from build123d import *

# Parameters (mm, degrees)
SKETCH1_R                           = 12.5
BOSS_EXTRUDE1_DEPTH                 = 50
CUT_EXTRUDE1_REACH                  = 55.033
CUT_EXTRUDE1_END_RADIUS             = 12.5
SKETCH2_R                           = 7
CUT_EXTRUDE1_DIRECTION_2_REACH      = 55.033
CUT_EXTRUDE1_DIRECTION_2_END_RADIUS = 12.5
CUT_EXTRUDE2_REACH                  = 55.033
SKETCH3_W                           = 9
SKETCH3_H                           = 20
CUT_EXTRUDE2_DIRECTION_2_REACH      = 55.033
SKETCH4_OUTSIDE_W                   = 48.214
SKETCH4_OUTSIDE_H                   = 48.214
SKETCH4_OUTSIDE_W_2                 = 17
SKETCH4_OUTSIDE_H_2                 = 17
CUT_EXTRUDE4_DEPTH                  = 30
SKETCH5_R                           = 12.5
SKETCH5_R_2                         = 7.5
CUT_EXTRUDE5_DEPTH                  = 70
CHAMFER2_SIZE                       = 2.5
CHAMFER1_SIZE                       = 0.25
SKETCH7_R                           = 12.5
BOSS_EXTRUDE2_DEPTH                 = 5


with BuildPart() as part:
    # Sketch1 → Boss-Extrude1 (new, symmetric)
    with BuildSketch(Plane(origin=(0, 0, 0), x_dir=(1, 0, 0), z_dir=(0, 1, 0))):
        with Locations(Location((0, 0, 0), (0, 0, 270))):
            Circle(SKETCH1_R)
    extrude(amount=BOSS_EXTRUDE1_DEPTH, both=True)

    # Cut-Extrude1: up to this cylinder (the profile starts inside it)
    cut_extrude1_end = Plane(origin=(0, -42, 0), z_dir=(0, -1, 0)) * Cylinder(CUT_EXTRUDE1_END_RADIUS, 136.066, mode=Mode.PRIVATE)
    # Sketch2 → Cut-Extrude1 (cut, up to the surface)
    with BuildSketch(Plane.XY, mode=Mode.PRIVATE) as cut_extrude1_sk1:
        with Locations(Location((0, -42, 0), (0, 0, 180))):
            Circle(SKETCH2_R)
    cut_extrude1_tool1 = extrude(cut_extrude1_sk1.sketch, amount=-CUT_EXTRUDE1_REACH, mode=Mode.PRIVATE) & cut_extrude1_end
    add(cut_extrude1_tool1.solids().sort_by_distance((0, -42, 0))[0], mode=Mode.SUBTRACT)

    # Cut-Extrude1 direction 2: up to this cylinder (the profile starts inside it)
    cut_extrude1_direction_2_end = Plane(origin=(0, -42, 0), z_dir=(0, -1, 0)) * Cylinder(CUT_EXTRUDE1_DIRECTION_2_END_RADIUS, 136.066, mode=Mode.PRIVATE)
    # Sketch2 → Cut-Extrude1 direction 2 (cut, up to the surface)
    with BuildSketch(Plane.XY, mode=Mode.PRIVATE) as cut_extrude1_direction_2_sk1:
        with Locations(Location((0, -42, 0), (0, 0, 180))):
            Circle(SKETCH2_R)
    cut_extrude1_direction_2_tool1 = extrude(cut_extrude1_direction_2_sk1.sketch, amount=CUT_EXTRUDE1_DIRECTION_2_REACH, mode=Mode.PRIVATE) & cut_extrude1_direction_2_end
    add(cut_extrude1_direction_2_tool1.solids().sort_by_distance((0, -42, 0))[0], mode=Mode.SUBTRACT)

    # Sketch3 → Cut-Extrude2 (cut, up to next)
    with BuildSketch(Plane(origin=(0, 0, 0), x_dir=(0, 0, -1), z_dir=(1, 0, 0)), mode=Mode.PRIVATE) as cut_extrude2_sk1:
        with Locations((0, -40)):
            Rectangle(SKETCH3_W, SKETCH3_H)
    cut_extrude2_tool1 = extrude(cut_extrude2_sk1.sketch, amount=-CUT_EXTRUDE2_REACH, mode=Mode.PRIVATE) & part.part
    add(cut_extrude2_tool1.solids().sort_by_distance((0, -40, 0))[0], mode=Mode.SUBTRACT)

    # Sketch3 → Cut-Extrude2 direction 2 (cut, up to next)
    with BuildSketch(Plane(origin=(0, 0, 0), x_dir=(0, 0, -1), z_dir=(1, 0, 0)), mode=Mode.PRIVATE) as cut_extrude2_direction_2_sk1:
        with Locations((0, -40)):
            Rectangle(SKETCH3_W, SKETCH3_H)
    cut_extrude2_direction_2_tool1 = extrude(cut_extrude2_direction_2_sk1.sketch, amount=CUT_EXTRUDE2_DIRECTION_2_REACH, mode=Mode.PRIVATE) & part.part
    add(cut_extrude2_direction_2_tool1.solids().sort_by_distance((0, -40, 0))[0], mode=Mode.SUBTRACT)

    # Sketch4 outside → Cut-Extrude4 (cut)
    with BuildSketch(Plane.XZ.offset(50)):
        Rectangle(SKETCH4_OUTSIDE_W, SKETCH4_OUTSIDE_H)
        Rectangle(SKETCH4_OUTSIDE_W_2, SKETCH4_OUTSIDE_H_2, mode=Mode.SUBTRACT)
    extrude(amount=-CUT_EXTRUDE4_DEPTH, mode=Mode.SUBTRACT)

    # Sketch5 → Cut-Extrude5 (cut)
    with BuildSketch(Plane(origin=(0, 50, 0), x_dir=(1, 0, 0), z_dir=(0, 1, 0))):
        Circle(SKETCH5_R)
        with Locations(Location((0, 0, 0), (0, 0, 270))):
            Circle(SKETCH5_R_2, mode=Mode.SUBTRACT)
    extrude(amount=-CUT_EXTRUDE5_DEPTH, mode=Mode.SUBTRACT)

    # Chamfer2
    chamfer2_edges = [part.edges().sort_by_distance(p)[0] for p in [
        (8.5, -50, 6.5),
        (8.5, -50, -6.5),
        (-8.5, -50, 6.5),
        (-8.5, -50, -6.5),
    ]]
    chamfer(chamfer2_edges, length=CHAMFER2_SIZE)

    # Chamfer1
    chamfer1_edges = [part.edges().sort_by_distance(p)[0] for p in [
        (-8.5, -30, 0),
        (8.5, -30, 0),
        (0, -20, -8.5),
        (8.5, -20, 0),
        (0, -20, 8.5),
        (-8.5, -20, 0),
        (8.5, -38.75, 4.5),
        (8.5, -33.75, -8.5),
        (-8.5, -33.75, -8.5),
        (-8.5, -38.75, -4.5),
        (-8.5, -33.75, 8.5),
        (8.5, -33.75, 8.5),
        (0, -50, -4.5),
        (0, -50, -8.5),
        (8.5, -38.75, -4.5),
        (-7.25, -48.75, -4.5),
        (7.25, -48.75, -4.5),
        (-7.25, -48.75, -8.5),
        (7.25, -48.75, -8.5),
        (0, -50, 8.5),
        (0, -50, 4.5),
        (-7.25, -48.75, 8.5),
        (7.25, -48.75, 8.5),
        (-8.5, -38.75, 4.5),
        (-7.25, -48.75, 4.5),
        (7.25, -48.75, 4.5),
    ]]
    chamfer(chamfer1_edges, length=CHAMFER1_SIZE)

    # Sketch7 → Boss-Extrude2 (add)
    with BuildSketch(Plane(origin=(0, -20, 0), x_dir=(1, 0, 0), z_dir=(0, 1, 0))):
        with Locations(Location((0, 0, 0), (0, 0, 270))):
            Circle(SKETCH7_R)
    extrude(amount=BOSS_EXTRUDE2_DEPTH)


solid = part.part
Can you work these out from the model? Positions are in its coordinate system, mm. A direction names the side the tool comes from. Round coordinates to 2 decimals unless told otherwise and drop trailing zeros. Write each loop counter-clockwise with the first axis right and the second up, starting at its lowest first coordinate (ties: lowest second). Pieces come first, ordered by that corner, then holes. Notation, with made-up numbers: (10.5, 38) - (32.5, 38) arc R13 cw to (32.5, 61) - close; hole circle Ø10 at (10.25, 66). An arc over 180 degrees is marked (long way). Write each question's results on one line, items separated by ' | '. Start each with the question number.
1) We'd pull the mould along Z, two halves only. Please class faces 1 (the flat face through (7.18, -48.65, 8.37)), 2 (the flat face through (7.18, -48.65, 4.63)), 3 (the flat face through (-7, -49, -7)): released by +Z, released by -Z, zero draft, split by the parting line, or undercut.
2) For pin 1 Ø4 at (x, y) = (-5, -10) entering from -Z; pin 2 Ø12 at (x, y) = (2, 15.5) entering from +Z; pin 3 Ø2 at (x, y) = (3, 37) entering from +Z, each with a flat end and sliding along its axis, tell me the tip position at first contact or that it passes through.
3) Suppose I cut it at B-B (x = 0). Give the number of separate pieces and of enclosed holes in the cut face, and give its area (3 significant figures).
4) Suppose I cut it at C-C (z = 0). List the corners of the cut face in (x, y) for me, and give its area (3 significant figures).
5) Which directions (+Z, -Z, +X, -X, +Y, -Y) give clear straight access to the entire face, cutting with the end or side of a thin tool? Please do faces 4 (the flat face through (0, -32, -8.5)), 5 (the flat face through (-8, -15, 0)), 6 (the flat face through (7.18, -48.64, -4.62)), 7 (the flat face through (-8.5, -28, 0)).
6) Suppose I cut it at A-A (y = -42). List the corners of the cut face in (x, z) for me, and give its area (4 significant figures).
7) Suppose I cut it at D-D (y = 31). List the corners of the cut face in (x, z) for me, and give its area (3 significant figures).
8) Please list where these lines run through material, in increasing order: line 1 (Y direction, x = 0, z = -6.8); line 2 (Y direction, x = -7.5, z = 9.75); line 3 (Z direction, x = 4.5, y = -9.5).
Here are the results:
1) face 1: released by +Z | face 2: undercut | face 3: zero draft
2) pin 1: stops at z = -6.87 | pin 2: stops at z = 7.5 | pin 3: stops at z = 7.23
3) separate pieces: 3 | enclosed holes: 0 | area: 1,320 mm2
4) outline: (-12.5, -20) - (-8.25, -20) - (-8.5, -20.25) - (-8.5, -29.75) - (-8.25, -30) - (8.25, -30) - (8.5, -29.75) - (8.5, -20.25) - (8.25, -20) - (12.5, -20) - (12.5, -15) - (7.5, -15) - (7.5, 50) - (-7.5, 50) - (-7.5, -15) - (-12.5, -15) - close | area: 1,270 mm2
5) face 4: -Z, +X, -X, -Y | face 5: +Y | face 6: +X, -Y | face 7: +Z, -Z, -X, -Y
6) outline: (-8.5, -8.25) - (-8.25, -8.5) - (-7, -8.5) - (-7, -4.5) - (-8.25, -4.5) - (-8.5, -4.75) - close; (-8.5, 4.75) - (-8.25, 4.5) - (-7, 4.5) - (-7, 8.5) - (-8.25, 8.5) - (-8.5, 8.25) - close; (7, -8.5) - (8.25, -8.5) - (8.5, -8.25) - (8.5, -4.75) - (8.25, -4.5) - (7, -4.5) - close; (7, 4.5) - (8.25, 4.5) - (8.5, 4.75) - (8.5, 8.25) - (8.25, 8.5) - (7, 8.5) - close | area: 23.75 mm2
7) outline: circle Ø15 at (0, 0) | area: 177 mm2
8) line 1: y = -50 to -49, -35 to 50 | line 2: y = -20 to -15 | line 3: z = -6 to 6
